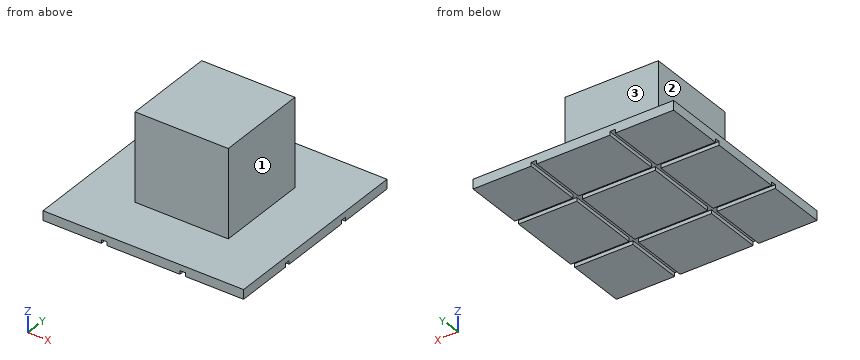
```python
from build123d import *

# Parameters (mm, degrees)
F0_W     = 6.477
F0_H     = 6.477
F1_DEPTH = 6.477
F4_START = 6.1214
F3_W     = 13.9445995965
F3_H     = 13.9445995965
F4_DEPTH = 0.6604
F5_W     = 0.381
F5_H     = 0.8794372982
F6_DEPTH = 12.7
F7_W     = 0.381
F7_H     = 1.3506091439
F8_DEPTH = 12.7
F9_ANGLE = 180


with BuildPart() as f1:
    # F0 (on Top) → F1 (new body)
    with BuildSketch(Plane.XY):
        with Locations((-9.8426504992, 11.6166997607)):
            Rectangle(F0_W, F0_H)
    extrude(amount=F1_DEPTH)


with BuildPart() as f1_1:
    # F2: moved
    add(f1.part.moved(Location((9.84707, -11.61667, 0))))

    # F3 (on Top) → F4 (join)
    with BuildSketch(Plane.XY.offset(F4_START)):
        with Locations((0.0044195008, 2.97607e-05)):
            Rectangle(F3_W, F3_H)
    extrude(amount=F4_DEPTH)

    # F5 (on Front) → F6 (cut, symmetric)
    with BuildSketch(Plane.XZ):
        with Locations((-2.7305, 6.9675186491)):
            Rectangle(F5_W, F5_H)
        with Locations((2.7305, 6.9675186491)):
            Rectangle(F5_W, F5_H)
    extrude(amount=F6_DEPTH, both=True, mode=Mode.SUBTRACT)

    # F7 (on Right) → F8 (cut, symmetric)
    with BuildSketch(Plane.YZ):
        with Locations((-2.7305, 7.203104572)):
            Rectangle(F7_W, F7_H)
        with Locations((2.7305, 7.203104572)):
            Rectangle(F7_W, F7_H)
    extrude(amount=F8_DEPTH, both=True, mode=Mode.SUBTRACT)


with BuildPart() as f1_2:
    # F9: moved
    add(f1_1.part.rotate(Axis((-3.2340804992, 2.97607e-05, 0), (0, -1, 0)), F9_ANGLE))


solid = f1_2.part
```
Input: part model. Units: mm. Frame: model coordinates. Face numbers are marked on the shaded views. A direction names the side the tool comes from. Coordinates: 2 decimals unless noted, no trailing zeros. Write each loop counter-clockwise with the first axis right and the second up, starting at its lowest first coordinate (ties: lowest second). Pieces come first, ordered by that corner, then holes. Notation, with made-up numbers: (76.5, 81.25) -> (123.5, 81.25) arc R24 cw to (123.5, 108.25) -> close; hole circle Ø8 at (34, 4). An arc over 180 degrees is marked (long way). Write each question's results on one line, items separated by ' | '.
Item 1: Section query A-A on x = -12. Return loops of the section in (y, z).
Conclusion:
outline: (-6.97, -6.78) -> (-2.92, -6.78) -> (-2.92, -6.53) -> (-2.54, -6.53) -> (-2.54, -6.78) -> (2.54, -6.78) -> (2.54, -6.53) -> (2.92, -6.53) -> (2.92, -6.78) -> (6.97, -6.78) -> (6.97, -6.12) -> (-6.97, -6.12) -> close
Item 2: Pin query (flat end, axial travel): pin 1 Ø3 at (y, z) = (4.5, -2) entering from +X; pin 2 Ø1.8 at (x, z) = (-6, -3) entering from -Y; pin 3 Ø5 at (x, y) = (-3, -3.5) entering from +Z. Return the tip coordinate at first contact, or that it passes through.
Conclusion:
pin 1: stops at x = -3.23 | pin 2: stops at y = -3.24 | pin 3: stops at z = 0
Item 3: Set-up query: the marked faces 1, 2 and 3. Return all of +Z, -Z, +X, -X, +Y, -Y with unobstructed straight access to the full face (end or side cutting, diameter ignored); none if empty.
Conclusion:
face 1: +Z, +X, +Y, -Y | face 2: +Z, -X, +Y, -Y | face 3: +Z, +X, -X, +Y
Item 4: Section query B-B on y = 2.75. Return loops of the section in (x, z).
Conclusion:
outline: (-13.44, -6.53) -> (0.5, -6.53) -> (0.5, -6.12) -> (-3.23, -6.12) -> (-3.23, 0) -> (-9.71, 0) -> (-9.71, -6.12) -> (-13.44, -6.12) -> close
Item 5: Section query C-C on z = -0.75. Return loops of the section in (x, y).
Conclusion:
outline: (-9.71, -3.24) -> (-3.23, -3.24) -> (-3.23, 3.24) -> (-9.71, 3.24) -> close
Item 6: Material intervals for probe 1 along X at (y, z) = (2.75, -5.5); probe 2 along Z at (x, y) = (-1.75, 1); probe 3 along Y at (x, z) = (-7.75, -4.5), sorted ascending.
Conclusion:
probe 1: x = -9.71 to -3.23 | probe 2: z = -6.78 to -6.12 | probe 3: y = -3.24 to 3.24
Item 7: Section query D-D on y = -3.5. Return loops of the section in (x, z), plus the area to 3 significant figures.
Conclusion:
outline: (-13.44, -6.78) -> (-9.39, -6.78) -> (-9.39, -6.53) -> (-9.01, -6.53) -> (-9.01, -6.78) -> (-3.93, -6.78) -> (-3.93, -6.53) -> (-3.55, -6.53) -> (-3.55, -6.78) -> (0.5, -6.78) -> (0.5, -6.12) -> (-13.44, -6.12) -> close | area: 9.02 mm^2
